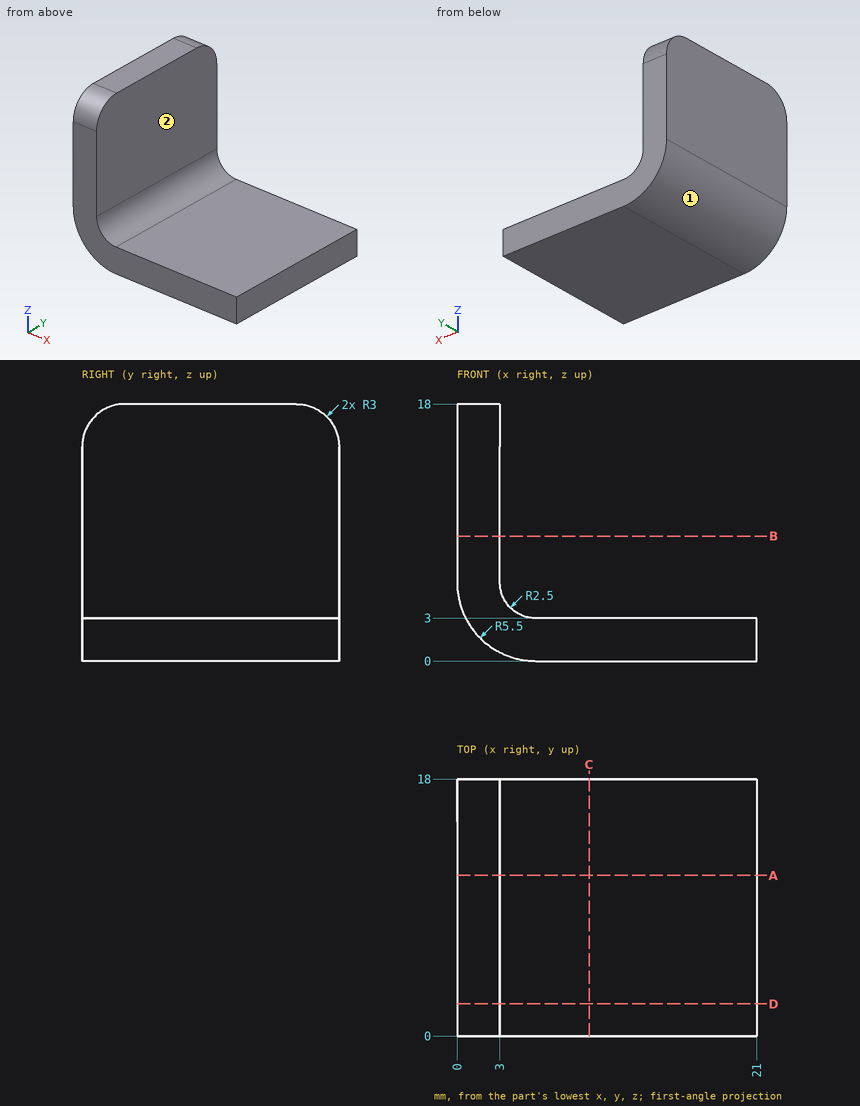
Design review of the part shown in the three views and the two pictorial views. Dimensions are in mm from the part's minimum x, y and z. A direction names the side the tool comes from. Give positions to 0.01 mm unless a question says otherwise; leave off trailing zeros. Loops run counter-clockwise (first coordinate to the right, second up) from the corner with the lowest first, then second, coordinate; pieces in that order, holes last. Notation, with made-up numbers: (70.25, 51) -> (128.25, 51) arc R31 cw to (128.25, 79) -> close; hole circle Ø11 at (-9.75, -22.75). An arc over 180 degrees is marked (long way). Write each question's results on one line, items separated by ' | '.
1) Take a section at D-D, the plane y = 2.25. Give the boundary of the cut face in (x, z).
Conclusion:
outline: (0, 5.5) arc R5.5 ccw to (5.5, 0) -> (21, 0) -> (21, 3) -> (5.5, 3) arc R2.5 cw to (3, 5.5) -> (3, 17.9) -> (0, 17.9) -> close
2) Take a section at C-C, the plane x = 9.25. Give the boundary of the cut face in (y, z).
Conclusion:
outline: (0, 0) -> (18, 0) -> (18, 3) -> (0, 3) -> close
3) Take a section at B-B, the plane z = 8.75. Give the boundary of the cut face in (x, y).
Conclusion:
outline: (0, 0) -> (3, 0) -> (3, 18) -> (0, 18) -> close
4) For line 1 along Z through (x, y) = (6, 8.75); line 2 along X through (y, z) = (6.5, 1.5), list the stretches that pass through material, from the lowest coordinate up. Write a range as from..to.
Conclusion:
line 1: z = 0..3 | line 2: x = 1.73..21
5) Tool access review of the marked faces 1 and 2: name each direction out of +Z, -Z, +X, -X, +Y, -Y from which nothing blocks a thin tool from reaching the whole face with its end or side.
Conclusion:
face 1: -Z, -X, +Y, -Y | face 2: +Z, +X, +Y, -Y
6) Take a section at A-A, the plane y = 11.25. Give the boundary of the cut face in (x, z).
Conclusion:
outline: (0, 5.5) arc R5.5 ccw to (5.5, 0) -> (21, 0) -> (21, 3) -> (5.5, 3) arc R2.5 cw to (3, 5.5) -> (3, 18) -> (0, 18) -> close
7) Insertion check: pin 1 Ø4 at (y, z) = (12.5, 10) entering from +X; pin 2 Ø4.5 at (x, y) = (16, 9.5) entering from +Z. Each pin has a flat end and moves straight along its axis. Give the tip position at first contact, or say it passes through.
Conclusion:
pin 1: stops at x = 3 | pin 2: stops at z = 3
